```python
from build123d import *

# Parameters (mm, degrees)
SKETCH1_W           = 60
SKETCH1_H           = 42
BOSS_EXTRUDE1_DEPTH = 5
SKETCH2_W           = 50
SKETCH2_H           = 32
CUT_EXTRUDE1_DEPTH  = 5
FILLET1_R           = 2.5
FILLET2_R           = 2.5


with BuildPart() as part:
    # Sketch1 → Boss-Extrude1 (new body)
    with BuildSketch(Plane(origin=(0, 0, 0), x_dir=(1, 0, 0), z_dir=(0, 1, 0))):
        with Locations((-3.018867925, 4.471698113)):
            Rectangle(SKETCH1_W, SKETCH1_H)
    extrude(amount=BOSS_EXTRUDE1_DEPTH)

    # Sketch2 → Cut-Extrude1 (cut)
    with BuildSketch(Plane(origin=(0, 5, 0), x_dir=(1, 0, 0), z_dir=(0, 1, 0))):
        with Locations((-3.018867925, 4.471698113)):
            Rectangle(SKETCH2_W, SKETCH2_H)
    extrude(amount=-CUT_EXTRUDE1_DEPTH, mode=Mode.SUBTRACT)

    # Fillet1
    fillet1_edges = [part.edges().sort_by_distance(p)[0] for p in [
        (-3.018867925, 5, 16.528301887),
        (-33.018867925, 5, -4.471698113),
        (-28.018867925, 5, -4.471698113),
        (-3.018867925, 5, 11.528301887),
        (21.981132075, 5, -4.471698113),
        (-3.018867925, 5, -20.471698113),
        (-3.018867925, 5, -25.471698113),
        (26.981132075, 5, -4.471698113),
    ]]
    fillet(fillet1_edges, radius=FILLET1_R - 0.0001)  # a hair under: the kernel refuses the full size

    # Fillet2
    fillet2_edges = [part.edges().sort_by_distance(p)[0] for p in [
        (-33.018867925, 0, -4.471698113),
        (-3.018867925, 0, 16.528301887),
        (26.981132075, 0, -4.471698113),
        (-3.018867925, 0, -25.471698113),
        (-3.018867925, 0, -20.471698113),
        (21.981132075, 0, -4.471698113),
        (-3.018867925, 0, 11.528301887),
        (-28.018867925, 0, -4.471698113),
    ]]
    fillet(fillet2_edges, radius=FILLET2_R - 0.0001)  # a hair under: the kernel refuses the full size


solid = part.part
```
Input: part model. Units: mm. Frame: model coordinates. A direction names the side the tool comes from. Coordinates: 2 decimals unless noted, no trailing zeros. Loops run counter-clockwise (first coordinate to the right, second up) from the corner with the lowest first, then second, coordinate; pieces in that order, holes last. Notation, with made-up numbers: (-25.5, 75.5) -> (-6.5, 75.5) arc R23 ccw to (-6.5, 95.5) -> close; hole circle Ø11 at (35, 49). An arc over 180 degrees is marked (long way). Use a Markdown table: item, result.
1) Access query for faces 1 (the cylindrical face through (-2.634, 0.713, -21.223)), 2 (the cylindrical face through (22.733, 4.287, -4.731)), 3 (the cylindrical face through (-2.599, 4.248, 15.815)). Directions: +Z, -Z, +X, -X, +Y, -Y. A direction counts if a zero-diameter tool reaches every point of the face in a straight line with its end or side. Return the directions, or none.
Results found:
| item | result |
|---|---|
| face 1 | -Y |
| face 2 | +Y |
| face 3 | +Z, +X, -X, +Y |
2) Material intervals for line 1 along Z through (x, y) = (12.5, 2.3); line 2 along X through (y, z) = (4.2, -3); line 3 along Z through (x, y) = (1.5, 4.6), sorted ascending. Write a range as from..to.
Results found:
| item | result |
|---|---|
| line 1 | z = -25.46..-20.48, 11.54..16.52 |
| line 2 | x = -32.35..-28.69, 22.65..26.31 |
| line 3 | z = -24.33..-21.62, 12.67..15.38 |
3) Cut plane C-C (y = 1.4). Return the cut outline in (x, z).
Results found:
| item | result |
|---|---|
| outline | (-32.76, -25.22) -> (26.73, -25.22) -> (26.73, 16.27) -> (-32.76, 16.27) -> close; hole (-28.27, -20.73) -> (22.24, -20.73) -> (22.24, 11.78) -> (-28.27, 11.78) -> close |
4) Pull-direction query (Z, two-part tool) for faces 4 (the cylindrical face through (-32.306, 0.752, -4.766)), 5 (the cylindrical face through (22.733, 0.713, -4.731)), 6 (the cylindrical face through (-2.599, 0.752, 15.815)); classes: released by +Z, released by -Z, zero draft, split by the parting line, or undercut.
Results found:
| item | result |
|---|---|
| face 4 | zero draft |
| face 5 | undercut |
| face 6 | released by +Z |
